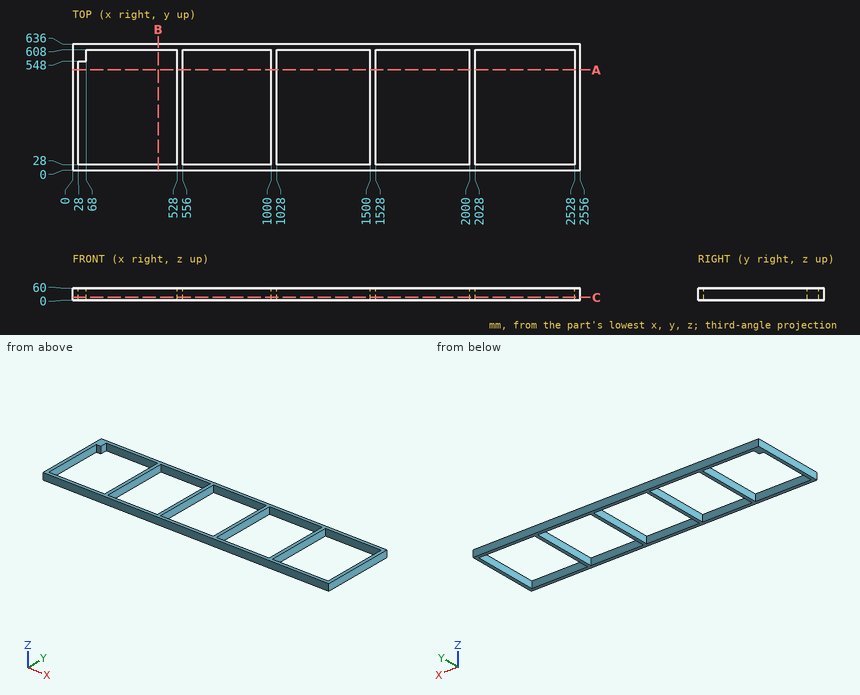
Study the drawing (mm; zero at the part's minimum x, y, z) and answer. Round coordinates to 2 decimals unless told otherwise and drop trailing zeros. Write each loop counter-clockwise with the first axis right and the second up, starting at its lowest first coordinate (ties: lowest second). Pieces come first, ordered by that corner, then holes.
1) A cutting plane is placed at C-C on z = 14. Determine the outline of the cut face in (x, y).
2) A cutting plane is placed at B-B on x = 431. Determine the outline of the cut face in (y, z).
3) Consider probe 1 along X at (y, z) = (124, 38); probe 2 along Y at (x, z) = (1178, 37). Determine where each line is inside the solid, lowest interval first.
4) A cutting plane is placed at A-A on y = 505.5. Determine the outline of the cut face in (x, z), and give its area (3 significant figures).
Entries:
1. outline: (0, 0) - (2556, 0) - (2556, 636) - (0, 636) - close; hole (28, 28) - (528, 28) - (528, 608) - (68, 608) - (68, 548) - (28, 548) - close; hole (556, 28) - (1000, 28) - (1000, 608) - (556, 608) - close; hole (1028, 28) - (1500, 28) - (1500, 608) - (1028, 608) - close; hole (1528, 28) - (2000, 28) - (2000, 608) - (1528, 608) - close; hole (2028, 28) - (2528, 28) - (2528, 608) - (2028, 608) - close
2. outline: (0, 0) - (28, 0) - (28, 60) - (0, 60) - close; (608, 0) - (636, 0) - (636, 60) - (608, 60) - close
3. probe 1: x = 0 to 28, 528 to 556, 1000 to 1028, 1500 to 1528, 2000 to 2028, 2528 to 2556
3. probe 2: y = 0 to 28, 608 to 636
4. outline: (0, 0) - (28, 0) - (28, 60) - (0, 60) - close; (528, 0) - (556, 0) - (556, 60) - (528, 60) - close; (1000, 0) - (1028, 0) - (1028, 60) - (1000, 60) - close; (1500, 0) - (1528, 0) - (1528, 60) - (1500, 60) - close; (2000, 0) - (2028, 0) - (2028, 60) - (2000, 60) - close; (2528, 0) - (2556, 0) - (2556, 60) - (2528, 60) - close
4. area: 10,100 mm2
